```python
from build123d import *

# Parameters (mm, degrees)
SKETCH1_W                 = 8.5
SKETCH1_H                 = 56.8
BOSS_EXTRUDE1_DEPTH       = 4.75
F_3_0MM_DOWEL_HOLE1_D     = 3
F_3_0MM_DOWEL_HOLE1_DEPTH = 5
F_3_0MM_DOWEL_HOLE1_TIP   = 0.901290929
SKETCH6_R                 = 2.85
CUT_EXTRUDE1_DEPTH        = 2.2


with BuildPart() as part:
    # Sketch1 → Boss-Extrude1 (new body)
    with BuildSketch(Plane.XY):
        with Locations((4.25, -28.4)):
            Rectangle(SKETCH1_W, SKETCH1_H)
    extrude(amount=BOSS_EXTRUDE1_DEPTH)

    # Ø3.0mm Dowel Hole1
    with Locations(Plane.XY.offset(4.75)):
        with Locations((4.25, -16.7), (4.25, -40.1)):
            Hole(F_3_0MM_DOWEL_HOLE1_D / 2, depth=F_3_0MM_DOWEL_HOLE1_DEPTH)
            with Locations((0, 0, -(F_3_0MM_DOWEL_HOLE1_DEPTH + F_3_0MM_DOWEL_HOLE1_TIP / 2))):  # 118° drill point
                Cone(0, F_3_0MM_DOWEL_HOLE1_D / 2, F_3_0MM_DOWEL_HOLE1_TIP, mode=Mode.SUBTRACT)

    # Sketch6 → Cut-Extrude1 (cut)
    with BuildSketch(Plane.XY.offset(4.75)):
        with Locations((4.25, -16.7)):
            Circle(SKETCH6_R)
        with Locations((4.25, -40.1)):
            Circle(SKETCH6_R)
    extrude(amount=-CUT_EXTRUDE1_DEPTH, mode=Mode.SUBTRACT)


solid = part.part
```
Geometry check sheet. Reference: the model listing, model coordinates, mm. A direction names the side the tool comes from. Coordinates: 2 decimals unless noted, no trailing zeros. Order: outer loops, then holes, each group sorted by start corner. A loop starts at its lowest first (then second) coordinate and runs counter-clockwise, first axis right, second up.
Item 1: Scan lines: line 1 along Y through (x, z) = (4.25, 3.7); line 2 along Y through (x, z) = (4.25, 1.1); line 3 along Z through (x, y) = (6.5, -18). Record each from-to range of solid material in increasing order.
Item 2: Section check B-B (x = 4.25). Enter the section's corners in (y, z), plus the area to 3 significant figures.
Item 3: Mould release check, pull along Y, two halves, no side actions. Record for faces 1 (the flat face through (8.5, -29, 2)), 2 (the flat face through (4, 0, 2)), 3 (the flat face through (5.5, -41.3, 2.55)): released by +Y, released by -Y, zero draft, split by the parting line, or undercut.
Item 4: Section check C-C (z = 1). Enter the section's corners in (x, y), plus the area to 3 significant figures.
Item 5: Section check A-A (y = -16.7). Enter the section's corners in (x, z), plus the area to 3 significant figures.
Item 6: Tool access check on faces 4 (the cylindrical face through (5, -18, 1)), 5 (the cylindrical face through (5.565, -19.228, 3.665)). Record the directions out of +Z, -Z, +X, -X, +Y, -Y that give a thin tool (end or side, any length) a straight path to the whole face; none if there is none.
Item 7: Section check D-D (x = 2). Enter the section's corners in (y, z).
Item 8: Depth check by flat-ended pin: pin 1 (3.5 mm diameter, centred on x = 4.25, y = -40.1, fed in from +Z); pin 2 (2.5 mm diameter, centred on x = 4.25, y = -16.7, fed in from -Z). Enter the tip coordinate at first touch or a pass-through.
Check sheet entries:
1. line 1: y = -56.8 to -42.95, -37.25 to -19.55, -13.85 to 0
1. line 2: y = -56.8 to -41.6, -38.6 to -18.2, -15.2 to 0
1. line 3: z = 0 to 2.55
2. outline: (-56.8, 0) - (-41.6, 0) - (-41.6, 2.55) - (-42.95, 2.55) - (-42.95, 4.75) - (-56.8, 4.75) - close; (-38.6, 0) - (-18.2, 0) - (-18.2, 2.55) - (-19.55, 2.55) - (-19.55, 4.75) - (-37.25, 4.75) - (-37.25, 2.55) - (-38.6, 2.55) - close; (-15.2, 0) - (0, 0) - (0, 4.75) - (-13.85, 4.75) - (-13.85, 2.55) - (-15.2, 2.55) - close
2. area: 229 mm2
3. face 1: zero draft
3. face 2: released by +Y
3. face 3: undercut
4. outline: (0, -56.8) - (8.5, -56.8) - (8.5, 0) - (0, 0) - close; hole circle Ø3 at (4.25, -40.1); hole circle Ø3 at (4.25, -16.7)
4. area: 469 mm2
5. outline: (0, 0) - (2.75, 0) - (2.75, 2.55) - (1.4, 2.55) - (1.4, 4.75) - (0, 4.75) - close; (5.75, 0) - (8.5, 0) - (8.5, 4.75) - (7.1, 4.75) - (7.1, 2.55) - (5.75, 2.55) - close
5. area: 20.2 mm2
6. face 4: +Z, -Z
6. face 5: +Z
7. outline: (-56.8, 0) - (0, 0) - (0, 4.75) - (-14.95, 4.75) - (-14.95, 2.55) - (-18.45, 2.55) - (-18.45, 4.75) - (-38.35, 4.75) - (-38.35, 2.55) - (-41.85, 2.55) - (-41.85, 4.75) - (-56.8, 4.75) - close
8. pin 1: stops at z = 2.55
8. pin 2: passes through
